For this review, use the dimensioned drawing (mm, ordinates from the lowest corner) and the shaded views. Coordinates: 2 decimals unless noted, no trailing zeros. Loops run counter-clockwise (first coordinate to the right, second up) from the corner with the lowest first, then second, coordinate; pieces in that order, holes last. Notation, with made-up numbers: (28.5, -22.5) -> (32.5, -22.5) arc R19 ccw to (32.5, -6.5) -> close; hole circle Ø8 at (5.25, 64.5). An arc over 180 degrees is marked (long way). Use one line per item in the form item = value. Start each with the question number.
1. Consider section D-D (z = 20). State the section outline as (x, y) points, then the cut area to 3 significant figures.
2. For pin 1 (6 mm diameter, centred on x = 6.35, z = 6.35, fed in from +Y), flat-tipped, find the tip position at first contact; note if it passes through.
3. Consider section C-C (y = 4). State how many separate pieces and enclosed holes the cut face has, then the cut area to 3 significant figures.
4. Consider section A-A (x = 57.15). State the section outline as (y, z) points, then the cut area to 3 significant figures.
5. Wall thickness on line 1 (X direction, y = 4.25, z = 19.05); line 2 (Z direction, x = 57.15, y = 2.5); line 3 (X direction, y = 1.5, z = 116) (1 decimal): over which ranges is each line inside the solid? List them lowest first. Write a range as from..to.
6. Consider section B-B (z = 6.35). State the section outline as (x, y) points.
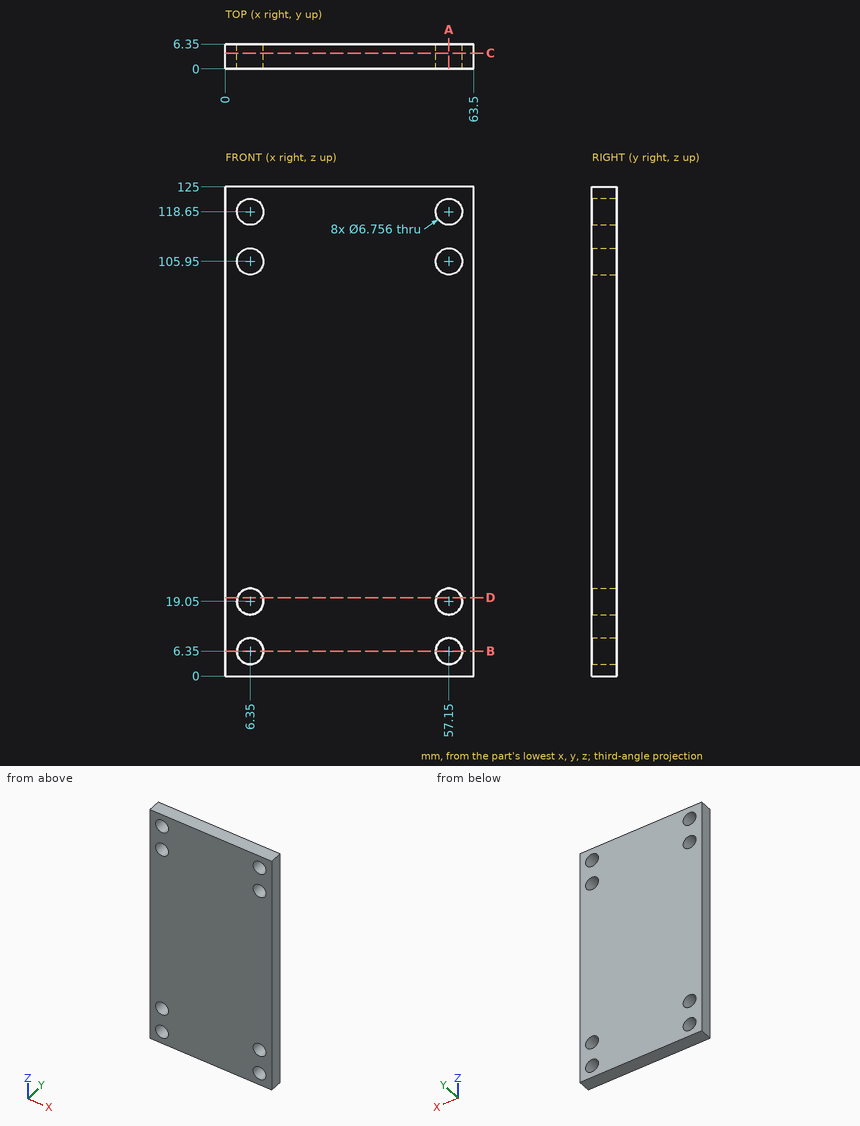
Geometry check:
q1.outline = (0, 0) -> (3.11, 0) -> (3.11, 6.35) -> (0, 6.35) -> close; (9.59, 0) -> (53.91, 0) -> (53.91, 6.35) -> (9.59, 6.35) -> close; (60.39, 0) -> (63.5, 0) -> (63.5, 6.35) -> (60.39, 6.35) -> close
q1.area = 321 mm²
q2.pin_1 = through
q3.separate_pieces = 1
q3.enclosed_holes = 8
q3.area = 7,650 mm²
q4.outline = (0, 0) -> (6.35, 0) -> (6.35, 2.97) -> (0, 2.97) -> close; (0, 9.73) -> (6.35, 9.73) -> (6.35, 15.67) -> (0, 15.67) -> close; (0, 22.43) -> (6.35, 22.43) -> (6.35, 102.57) -> (0, 102.57) -> close; (0, 109.33) -> (6.35, 109.33) -> (6.35, 115.27) -> (0, 115.27) -> close; (0, 122.03) -> (6.35, 122.03) -> (6.35, 125) -> (0, 125) -> close
q4.area = 622 mm²
q5.line_1 = 0..2.97, 9.73..53.77, 60.53..63.5
q5.line_2 = 0..2.97, 9.73..15.67, 22.43..102.57, 109.33..115.27, 122.03..125
q5.line_3 = 0..4.3, 8.4..55.1, 59.2..63.5
q6.outline = (0, 0) -> (2.97, 0) -> (2.97, 6.35) -> (0, 6.35) -> close; (9.73, 0) -> (53.77, 0) -> (53.77, 6.35) -> (9.73, 6.35) -> close; (60.53, 0) -> (63.5, 0) -> (63.5, 6.35) -> (60.53, 6.35) -> close
